Source: CAD feature listing. Evaluate the final solid. Frame: model axes, mm. A direction names the side the tool comes from. Coordinates: 2 decimals unless noted, no trailing zeros. Loops run counter-clockwise (first coordinate to the right, second up) from the corner with the lowest first, then second, coordinate; pieces in that order, holes last. Notation, with made-up numbers: (27, 57) -> (56, 57) arc R18 ccw to (56, 78) -> close; hole circle Ø10 at (62, -37). An arc over 180 degrees is marked (long way). One line per question, with ' | ' between items. Start each with the question number.
```python
from build123d import *

# Parameters (mm, degrees)
SKETCH_W        = 75
SKETCH_H        = 75
PAD_DEPTH       = 7
SKETCH001_R     = 1.4
PAD001_DEPTH    = 3
SKETCH002_W     = 41
SKETCH002_H     = 50
POCKET_DEPTH    = 5
SKETCH003_W     = 18
SKETCH003_H     = 22
POCKET001_DEPTH = 1
SKETCH004_W     = 18
SKETCH004_H     = 3.2
POCKET002_DEPTH = 6.001
SKETCH005_R     = 1.25
PAD002_DEPTH    = 3
SKETCH006_W     = 32
SKETCH006_H     = 10
POCKET003_DEPTH = 7.001


with BuildPart() as part:
    # Sketch → Pad (new body)
    with BuildSketch(Plane.XY):
        with Locations((37.5, 37.5)):
            Rectangle(SKETCH_W, SKETCH_H)
    extrude(amount=PAD_DEPTH)

    # Sketch001 (on Face6 of Pad) → Pad001 (join)
    with BuildSketch(Plane.XY.offset(7)):
        with Locations((5, 68)):
            Circle(SKETCH001_R)
        with Locations((45, 68)):
            Circle(SKETCH001_R)
        with Locations((5, 13)):
            Circle(SKETCH001_R)
        with Locations((45, 13)):
            Circle(SKETCH001_R)
    extrude(amount=PAD001_DEPTH)

    # Sketch002 (on Face5 of Pad001) → Pocket (cut)
    with BuildSketch(Plane.XY.offset(7)):
        with Locations((25.5, 40)):
            Rectangle(SKETCH002_W, SKETCH002_H)
    extrude(amount=-POCKET_DEPTH, mode=Mode.SUBTRACT)

    # Sketch003 (on Face5 of Pocket) → Pocket001 (cut)
    with BuildSketch(Plane.XY.offset(7)):
        with Locations((62.979134, 54)):
            Rectangle(SKETCH003_W, SKETCH003_H)
    extrude(amount=-POCKET001_DEPTH, mode=Mode.SUBTRACT)

    # Sketch004 (on Face23 of Pocket001) → Pocket002 (cut, through all)
    with BuildSketch(Plane.XY.offset(6)):
        with Locations((62.979134, 44.6)):
            Rectangle(SKETCH004_W, SKETCH004_H)
    extrude(amount=-POCKET002_DEPTH, mode=Mode.SUBTRACT)

    # Sketch005 (on Face23 of Pocket002) → Pad002 (join)
    with BuildSketch(Plane.XY.offset(6)):
        with Locations((55.979134, 61)):
            Circle(SKETCH005_R)
        with Locations((69.979134, 61)):
            Circle(SKETCH005_R)
    extrude(amount=PAD002_DEPTH)

    # Sketch006 (on Face5 of Pad002) → Pocket003 (cut, through all)
    with BuildSketch(Plane.XY.offset(7)):
        with Locations((26, 73)):
            Rectangle(SKETCH006_W, SKETCH006_H)
    extrude(amount=-POCKET003_DEPTH, mode=Mode.SUBTRACT)


solid = part.part
```
(1) Cut plane A-A, the plane x = 66. Return the cut outline in (y, z), and give its area (3 significant figures).
(2) Ray query, L1, parallel to X at y = 44.5, z = 4.75; L2, parallel to Y at x = 63, z = 4.5; L3, parallel to X at y = 17.5, z = 5. Return the intervals inside material, ascending.
(3) Draft query along X for faces 5 (the flat face through (71.979, 49.9, 6.4)), 6 (the flat face through (75, 37, 3)), 7 (the flat face through (5, 68, 10)). Return one class per face: pulls with the +X half, pulls with the -X half, needs draft (parallel to the pull), parting line crosses it, or undercut.
(4) Cut plane D-D, the plane x = 45. Return the cut outline in (y, z).
(5) Access query for faces 1 (the flat face through (63, 43, 4)), 2 (the flat face through (42, 71, 4)), 3 (the cylindrical face through (45.75, 14.18, 8.48)), 4 (the flat face through (5, 13, 10)). Directions: +Z, -Z, +X, -X, +Y, -Y. A direction counts if a zero-diameter tool reaches every point of the face in a straight line with its end or side. Return the directions, or none.
(6) Cut plane B-B, the plane z = 8. Return the cut outline in (x, y).
(7) Cut plane C-C, the plane y = 61. Return the cut outline in (x, z).
(8) Contact query for flat-ended pins moving along their axis: pin 1 Ø5.5 at (x, y) = (64.5, 54) entering from +Z; pin 2 Ø8 at (x, y) = (13.5, 37) entering from +Z; pin 3 Ø1.5 at (x, z) = (37.5, 2.5) entering from +Y. Output: stop coordinate, or through.
Here are the results:
1) outline: (0, 0) -> (43, 0) -> (43, 7) -> (0, 7) -> close; (46.2, 0) -> (75, 0) -> (75, 7) -> (65, 7) -> (65, 6) -> (46.2, 6) -> close | area: 484 mm2
2) L1: x = 0 to 5, 46 to 53.98, 71.98 to 75 | L2: y = 0 to 43, 46.2 to 75 | L3: x = 0 to 5, 46 to 75
3) face 5: undercut | face 6: pulls with the +X half | face 7: needs draft
4) outline: (0, 0) -> (75, 0) -> (75, 7) -> (69.4, 7) -> (69.4, 10) -> (66.6, 10) -> (66.6, 7) -> (65, 7) -> (65, 2) -> (15, 2) -> (15, 7) -> (14.4, 7) -> (14.4, 10) -> (11.6, 10) -> (11.6, 7) -> (0, 7) -> close
5) face 1: +Z, -Z | face 2: +Z, -Z, +Y | face 3: +Z | face 4: +Z, +X, -X, +Y, -Y
6) outline: circle Ø2.8 at (5, 13); circle Ø2.8 at (5, 68); circle Ø2.8 at (45, 13); circle Ø2.8 at (45, 68); circle Ø2.5 at (55.98, 61); circle Ø2.5 at (69.98, 61)
7) outline: (0, 0) -> (75, 0) -> (75, 7) -> (71.98, 7) -> (71.98, 6) -> (71.23, 6) -> (71.23, 9) -> (68.73, 9) -> (68.73, 6) -> (57.23, 6) -> (57.23, 9) -> (54.73, 9) -> (54.73, 6) -> (53.98, 6) -> (53.98, 7) -> (46, 7) -> (46, 2) -> (5, 2) -> (5, 7) -> (0, 7) -> close
8) pin 1: stops at z = 6 | pin 2: stops at z = 2 | pin 3: stops at y = 68
